Geometry: see drawing. Coordinates: mm, zero at the bounding-box minimum. Give positions to 0.01 mm unless a question says otherwise; leave off trailing zeros. Write each loop counter-clockwise with the first axis right and the second up, starting at its lowest first coordinate (ties: lowest second). Pieces come first, ordered by that corner, then holes. Notation, with made-up numbers: (13.5, -29) -> (67.5, -29) arc R27 ccw to (67.5, -12) -> close; hole circle Ø11 at (17.5, 63). An arc over 180 degrees is marked (long way). Write item = value, one per line.
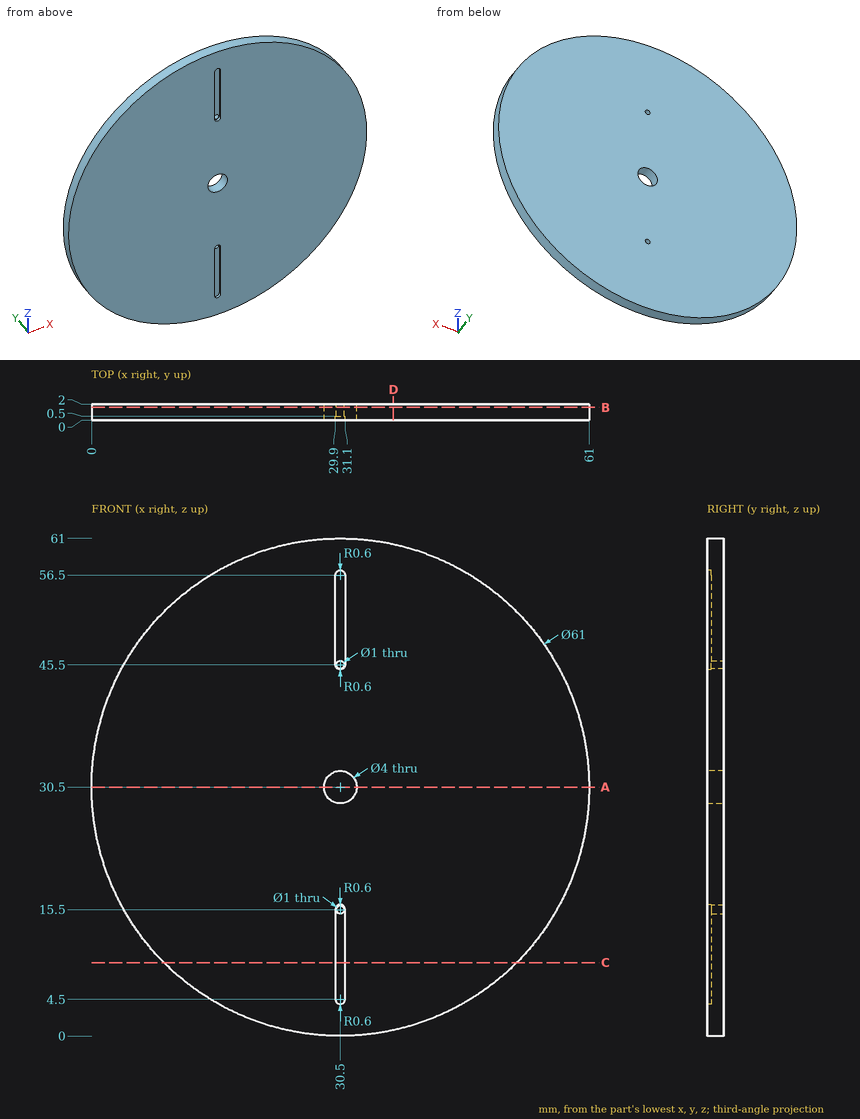
(1) Section query A-A (z = 30.5). Return loops of the section in (x, y), plus the area to 3 significant figures.
Values follow:
outline = (0, 0) -> (28.5, 0) -> (28.5, 2) -> (0, 2) -> close; (32.5, 0) -> (61, 0) -> (61, 2) -> (32.5, 2) -> close
area = 114 mm2
(2) Section query B-B (y = 1.6). Return loops of the section in (x, z), plus the area to 3 significant figures.
Values follow:
outline = circle Ø61 at (30.5, 30.5); hole circle Ø4 at (30.5, 30.5); hole circle Ø1 at (30.5, 15.5); hole circle Ø1 at (30.5, 45.5)
area = 2,910 mm2
(3) First-contact query: pin 1 (12 mm diameter, centred on x = 46.5, z = 35, fed in from -Y); pin 2 (0.6 mm diameter, centred on y = 0, z = 8.5, fed in from +X); pin 3 (0.6 mm diameter, centred on x = 30.5, z = 48.5, fed in from -Y). Flat tips, straight axial feed; report the tip coordinate or a pass-through.
Values follow:
pin_1 = 0
pin_2 = 51.93
pin_3 = 0.5
(4) Section query D-D (x = 37). Return loops of the section in (y, z).
Values follow:
outline = (0, 0.7) -> (2, 0.7) -> (2, 60.3) -> (0, 60.3) -> close
(5) Material intervals for line 1 (X direction, y = 1.4, z = 30.5); line 2 (X direction, y = 1, z = 15.5); line 3 (X direction, y = 1.05, z = 54.5), sorted ascending.
Values follow:
line_1 = 0 to 28.5, 32.5 to 61
line_2 = 3.94 to 30, 31 to 57.06
line_3 = 11.68 to 49.32
(6) Section query C-C (z = 9). Return loops of the section in (x, y).
Values follow:
outline = (8.87, 0) -> (29.9, 0) -> (29.9, 0.5) -> (31.1, 0.5) -> (31.1, 0) -> (52.13, 0) -> (52.13, 2) -> (8.87, 2) -> close
